Verification items for the finished model (mm, model axes). Round coordinates to 2 decimals unless told otherwise and drop trailing zeros. Order: outer loops, then holes, each group sorted by start corner. A loop starts at its lowest first (then second) coordinate and runs counter-clockwise, first axis right, second up. Notation, with made-up numbers: M -19,76 L 38,76 A20 cw 38,87 Z; hole C 60.5,-31 d9. An arc over 180 degrees is marked long. Use one line per item in the form item = value. Start each with the question number.
Item 1: Go/stop test with a flat-tipped pin: pin 1 Ø0.9 at (x, z) = (182.5, -3.5) entering from -Y. Record where the tip stops, or that it passes through.
Item 2: Cross-section at D-D on y = -1.85. Count the separate pieces of the cut face and the enclosed holes in it, then the cut area to 3 significant figures.
Item 3: Cross-section at A-A on x = 41.5. Enter the section's corners in (y, z).
Item 4: Thickness scan on probe 1 along Z at (x, y) = (182.5, -0.95); probe 2 along Z at (x, y) = (199.5, -1.95); probe 3 along X at (y, z) = (-1.7, -45). Record the ranges inside material, lowest first. Write a range as [from, to].
Item 5: Cross-section at C-C on x = 105. Enter the section's corners in (y, z).
Item 6: Cross-section at B-B on z = -24.5. Enter the section's corners in (x, y), then the cut area to 3 significant figures.
Autodesk Fusion 360 part; units mm, degrees
sketch "Skizze1" plane through (0, 0, 0) normal (0, 1, 0) x (1, 0, 0)
  line L0 (2, 0) -> (206, 0)
  line L1 (208, 2) -> (208, 109)
  line L2 (206, 111) -> (2, 111)
  line L3 (0, 109) -> (0, 2)
  circle A0 centre (8.575, 8.575) radius 1.5
  circle A1 centre (8.575, 102.425) radius 1.5
  circle A2 centre (199.425, 102.425) radius 1.5
  circle A3 centre (199.425, 8.575) radius 1.5
  line L4 (166.2, 106) -> (162.8, 106)
  line L5 (192, 106) -> (195.4, 106)
  line L6 (195.4, 89) -> (192, 89)
  line L7 (192, 68) -> (192, 76.4)
  line L8 (192, 76.4) -> (192, 71.4)
  line L9 (16.5, 77) -> (49.5, 77)
  line L10 (49.5, 77) -> (49.5, 44)
  line L11 (49.5, 44) -> (16.5, 44)
  line L12 (16.5, 44) -> (16.5, 77)
  line L13 (16.5, 77) -> (49.5, 77)
  line L14 (49.5, 77) -> (49.5, 74)
  line L15 (49.5, 74) -> (16.5, 74)
  line L16 (16.5, 74) -> (16.5, 77)
  line L17 (16.5, 74) -> (49.5, 74)
  line L18 (49.5, 74) -> (49.5, 71)
  line L19 (49.5, 71) -> (16.5, 71)
  line L20 (16.5, 71) -> (16.5, 74)
  line L21 (16.5, 71) -> (49.5, 71)
  line L22 (49.5, 71) -> (49.5, 68)
  line L23 (49.5, 68) -> (16.5, 68)
  line L24 (16.5, 68) -> (16.5, 71)
  line L25 (16.5, 68) -> (49.5, 68)
  line L26 (49.5, 68) -> (49.5, 65)
  line L27 (49.5, 65) -> (16.5, 65)
  line L28 (16.5, 65) -> (16.5, 68)
  line L29 (16.5, 65) -> (49.5, 65)
  line L30 (49.5, 65) -> (49.5, 62)
  line L31 (49.5, 62) -> (16.5, 62)
  line L32 (16.5, 62) -> (16.5, 65)
  line L33 (16.5, 62) -> (49.5, 62)
  line L34 (49.5, 62) -> (49.5, 59)
  line L35 (49.5, 59) -> (16.5, 59)
  line L36 (16.5, 59) -> (16.5, 62)
  line L37 (16.5, 59) -> (49.5, 59)
  line L38 (49.5, 59) -> (49.5, 56)
  line L39 (49.5, 56) -> (16.5, 56)
  line L40 (16.5, 56) -> (16.5, 59)
  line L41 (16.5, 56) -> (49.5, 56)
  line L42 (49.5, 56) -> (49.5, 53)
  line L43 (49.5, 53) -> (16.5, 53)
  line L44 (16.5, 53) -> (16.5, 56)
  line L45 (16.5, 53) -> (49.5, 53)
  line L46 (49.5, 53) -> (49.5, 50)
  line L47 (49.5, 50) -> (16.5, 50)
  line L48 (16.5, 50) -> (16.5, 53)
  line L49 (16.5, 50) -> (49.5, 50)
  line L50 (49.5, 50) -> (49.5, 47)
  line L51 (49.5, 47) -> (16.5, 47)
  line L52 (16.5, 47) -> (16.5, 50)
  line L53 (16.5, 47) -> (49.5, 47)
  line L54 (49.5, 47) -> (49.5, 44)
  line L55 (49.5, 44) -> (16.5, 44)
  line L56 (16.5, 44) -> (16.5, 47)
  line L57 (20, 109) -> (30.8, 109)
  line L58 (30.8, 109) -> (30.8, 106)
  line L59 (30.8, 106) -> (20, 106)
  line L60 (20, 106) -> (20, 109)
  line L61 (2, 91) -> (5, 91)
  line L62 (5, 91) -> (5, 80.2)
  line L63 (5, 80.2) -> (2, 80.2)
  line L64 (2, 80.2) -> (2, 91)
  line L65 (2, 30.8) -> (5, 30.8)
  line L66 (5, 30.8) -> (5, 20)
  line L67 (5, 20) -> (2, 20)
  line L68 (2, 20) -> (2, 30.8)
  line L69 (20, 5) -> (30.8, 5)
  line L70 (30.8, 5) -> (30.8, 2)
  line L71 (30.8, 2) -> (20, 2)
  line L72 (20, 2) -> (20, 5)
  line L73 (177.2, 5) -> (188, 5)
  line L74 (188, 5) -> (188, 2)
  line L75 (188, 2) -> (177.2, 2)
  line L76 (177.2, 2) -> (177.2, 5)
  line L77 (203, 30.8) -> (206, 30.8)
  line L78 (206, 30.8) -> (206, 20)
  line L79 (206, 20) -> (203, 20)
  line L80 (203, 20) -> (203, 30.8)
  line L81 (177.2, 109) -> (188, 109)
  line L82 (188, 109) -> (188, 106)
  line L83 (188, 106) -> (177.2, 106)
  line L84 (177.2, 106) -> (177.2, 109)
  line L85 (203, 91) -> (206, 91)
  line L86 (206, 91) -> (206, 80.2)
  line L87 (206, 80.2) -> (203, 80.2)
  line L88 (203, 80.2) -> (203, 91)
  line L89 (98.6, 5) -> (109.4, 5)
  line L90 (109.4, 5) -> (109.4, 2)
  line L91 (109.4, 2) -> (98.6, 2)
  line L92 (98.6, 2) -> (98.6, 5)
  line L93 (98.6, 109) -> (109.4, 109)
  line L94 (109.4, 109) -> (109.4, 106)
  line L95 (109.4, 106) -> (98.6, 106)
  line L96 (98.6, 106) -> (98.6, 109)
  line L97 (203, 60.9) -> (206, 60.9)
  line L98 (206, 60.9) -> (206, 50.1)
  line L99 (206, 50.1) -> (203, 50.1)
  line L100 (203, 50.1) -> (203, 60.9)
  line L101 (2, 60.9) -> (5, 60.9)
  line L102 (5, 60.9) -> (5, 50.1)
  line L103 (5, 50.1) -> (2, 50.1)
  line L104 (2, 50.1) -> (2, 60.9)
  arc A4 (2, 111) -> (0, 109) centre (2, 109) ccw
  arc A5 (0, 2) -> (2, 0) centre (2, 2) ccw
  arc A6 (206, 0) -> (208, 2) centre (206, 2) ccw
  arc A7 (208, 109) -> (206, 111) centre (206, 109) ccw
  circle A8 centre (118.425, 8.575) radius 1.5
  circle A9 centre (118.425, 102.425) radius 1.5
  point P0 (208, 0)
  point P1 (0, 111)
  dimension "d1" = 208
  dimension "d2" = 111
  dimension "d3" = 3
  dimension "d4" = 8.575
  dimension "d5" = 8.575
  dimension "d6" = 3
  dimension "d7" = 8.575
  dimension "d8" = 8.575
  dimension "d9" = 3
  dimension "d10" = 8.575
  dimension "d11" = 8.575
  dimension "d12" = 3
  dimension "d13" = 8.575
  dimension "d14" = 8.575
  dimension "d44" = 25.8
  dimension "d48" = 3.4
  dimension "d49" = 3.4
  dimension "d50" = 17
  dimension "d60" = 33
  dimension "d61" = 33
  dimension "d62" = 34
  dimension "d63" = 16.5
  dimension "d64" = 3
  dimension "d65" = 33
  dimension "d66" = 3
  dimension "d67" = 3
  dimension "d68" = 3
  dimension "d69" = 3
  dimension "d70" = 3
  dimension "d71" = 3
  dimension "d72" = 3
  dimension "d73" = 3
  dimension "d74" = 3
  dimension "d75" = 10.8
  dimension "d76" = 3
  dimension "d77" = 20
  dimension "d78" = 2
  dimension "d79" = 3
  dimension "d80" = 10.8
  dimension "d81" = 2
  dimension "d82" = 20
  dimension "d83" = 3
  dimension "d84" = 10.8
  dimension "d85" = 2
  dimension "d86" = 20
  dimension "d87" = 10.8
  dimension "d88" = 3
  dimension "d89" = 2
  dimension "d90" = 20
  dimension "d91" = 10.8
  dimension "d92" = 3
  dimension "d93" = 2
  dimension "d94" = 20
  dimension "d95" = 3
  dimension "d96" = 10.8
  dimension "d97" = 2
  dimension "d98" = 20
  dimension "d99" = 10.8
  dimension "d100" = 3
  dimension "d101" = 2
  dimension "d102" = 20
  dimension "d103" = 3
  dimension "d104" = 10.8
  dimension "d105" = 2
  dimension "d106" = 20
  dimension "d107" = 10.8
  dimension "d108" = 3
  dimension "d109" = 2
  dimension "d110" = 98.6
  dimension "d111" = 10.8
  dimension "d112" = 3
  dimension "d113" = 2
  dimension "d114" = 98.6
  dimension "d115" = 3
  dimension "d116" = 10.8
  dimension "d117" = 2
  dimension "d118" = 50.1
  dimension "d119" = 3
  dimension "d120" = 10.8
  dimension "d121" = 2
  dimension "d122" = 50.1
  dimension "d123" = 2
  dimension "d124" = 2
  dimension "d125" = 2
  dimension "d126" = 2
  dimension "d160" = 3
  dimension "d161" = 109.85
  dimension "d162" = 8.575
  dimension "d163" = 3
  dimension "d164" = 8.575
  dimension "d165" = 109.85
extrude "Extrusion11" add sketch "Skizze1" against normal blind 2.4 contours L0 L1 L2 L3 A4 A5 A6 A7 | L10 L12 L15 L17 L18 L19 L20 L21 | L10 L12 L23 L25 L26 L27 L28 L29 | L10 L12 L31 L33 L34 L35 L36 L37 | L10 L12 L39 L41 L42 L43 L44 L45 | L10 L12 L47 L49 L50 L51 L52 L53
extrude "Extrusion12" add sketch "Skizze1" against normal blind 0.6 contours L57 L58 L59 L60 | L61 L62 L63 L64 | L65 L66 L67 L68 | L69 L70 L71 L72 | L73 L74 L75 L76 | L77 L78 L79 L80 | L81 L82 L83 L84 | L85 L86 L87 L88 | L89 L90 L91 L92 | L93 L94 L95 L96 | L97 L98 L99 L100 | L101 L102 L103 L104
hole "Bohrung5" at (8.575, 0, -8.575) direction (0, -1, 0) diameter 6 depth 0.9 tip angle 180
hole "Bohrung6" at (8.575, 0, -102.425) direction (0, -1, 0) diameter 6 depth 0.9 tip angle 180
hole "Bohrung7" at (118.425, 0, -102.425) direction (0, -1, 0) diameter 6 depth 0.9 tip angle 180
hole "Bohrung8" at (118.425, 0, -8.575) direction (0, -1, 0) diameter 6 depth 0.9 tip angle 180
hole "Bohrung9" at (199.425, 0, -102.425) direction (0, -1, 0) diameter 6 depth 0.9 tip angle 180
hole "Bohrung10" at (199.425, 0, -8.575) direction (0, -1, 0) diameter 6 depth 0.9 tip angle 180
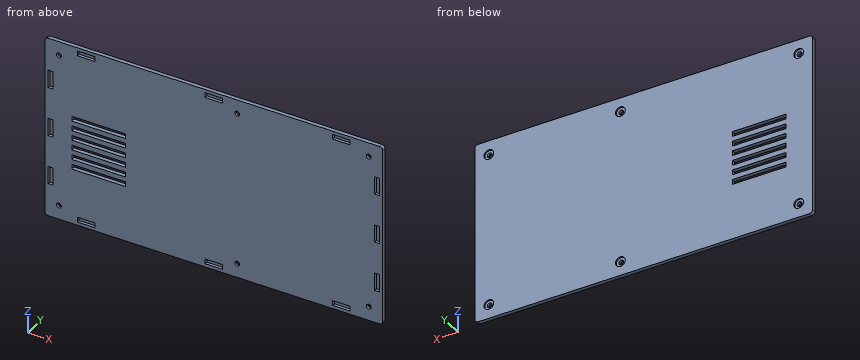
Output values:
q1.pin_1 = -0.6
q2.separate_pieces = 1
q2.enclosed_holes = 24
q2.area = 22,100 mm2
q3.outline = M -2.4,-111 L 0,-111 L 0,-77 L -2.4,-77 Z; M -2.4,-74 L 0,-74 L 0,-71 L -2.4,-71 Z; M -2.4,-68 L 0,-68 L 0,-65 L -2.4,-65 Z; M -2.4,-62 L 0,-62 L 0,-59 L -2.4,-59 Z; M -2.4,-56 L 0,-56 L 0,-53 L -2.4,-53 Z; M -2.4,-50 L 0,-50 L 0,-47 L -2.4,-47 Z; M -2.4,-44 L 0,-44 L 0,0 L -2.4,0 Z
q4.probe_1 = [-111, -109], [-106, -5], [-2, 0]
q4.probe_2 = [-111, -103.92], [-100.93, -10.07], [-7.08, 0]
q4.probe_3 = [0, 16.5], [49.5, 208]
q5.outline = M -2.4,-111 L 0,-111 L 0,0 L -2.4,0 L -2.4,-2 L -0.6,-2 L -0.6,-5 L -2.4,-5 L -2.4,-106 L -0.6,-106 L -0.6,-109 L -2.4,-109 Z
q6.outline = M 0,-2.4 L 2,-2.4 L 2,-0.6 L 5,-0.6 L 5,-2.4 L 203,-2.4 L 203,-0.6 L 206,-0.6 L 206,-2.4 L 208,-2.4 L 208,0 L 0,0 Z
q6.area = 488 mm2
